Can you work these out from the drawing? Everything is in mm from the part's minimum corner. A direction names the side the tool comes from. Round coordinates to 2 decimals unless told otherwise and drop trailing zeros. Loops run counter-clockwise (first coordinate to the right, second up) from the corner with the lowest first, then second, coordinate; pieces in that order, holes last. Notation, with made-up numbers: M -22.75,75.25 L -3.75,75.25 A32 cw -3.75,103.25 Z; hole C -4.75,11 d1. An arc over 180 degrees is marked long. Use a Markdown table: item, result.
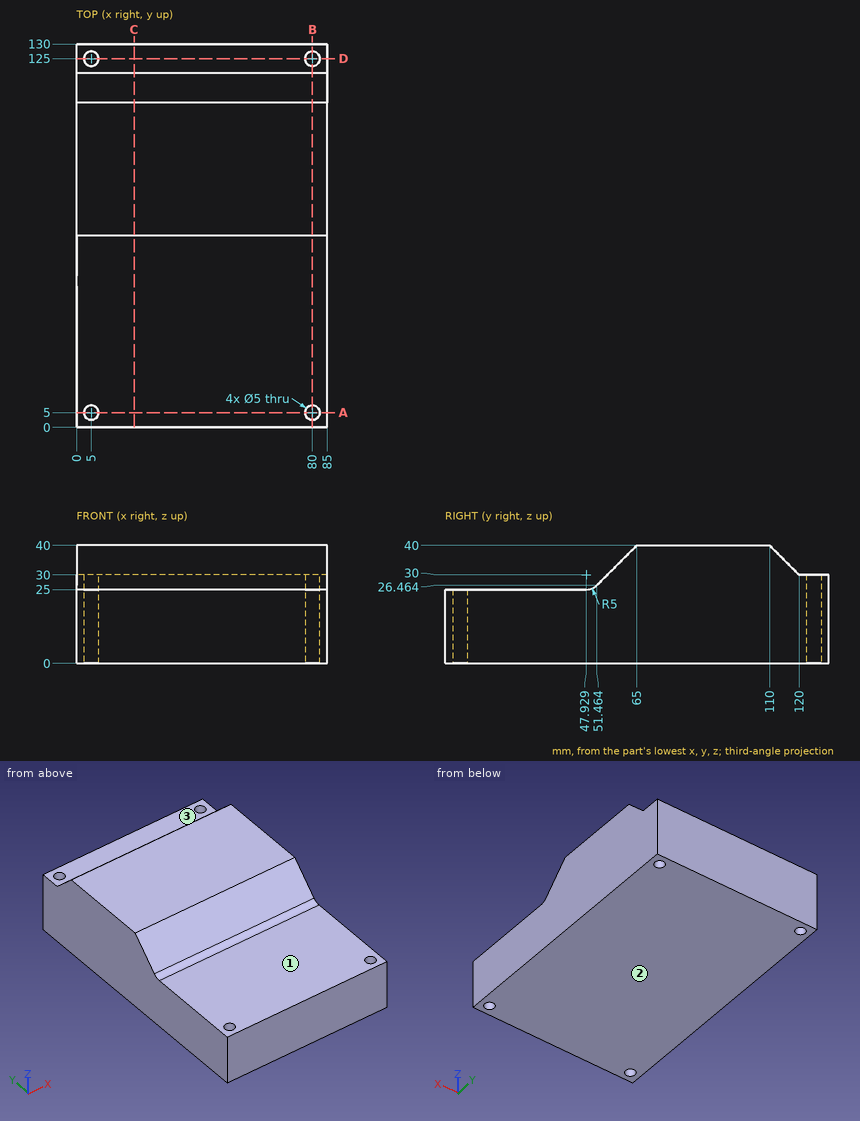
Q1. I need wall thicknesses on line 1 (Y direction, x = 80, z = 21); line 2 (X direction, y = 125, z = 16.5); line 3 (Y direction, x = 78.5, z = 19.5). Which ranges of each line are inside material? Lowest first, please. Write a range as from..to.
Return value:
| item | result |
|---|---|
| line 1 | y = 0..2.5, 7.5..122.5, 127.5..130 |
| line 2 | x = 0..2.5, 7.5..77.5, 82.5..85 |
| line 3 | y = 0..3, 7..123, 127..130 |
Q2. Imagine slicing it at C-C, the plane x = 19.5. Please give me the cut outline in (y, z) (1 decimal).
Return value:
| item | result |
|---|---|
| outline | M 0,0 L 130,0 L 130,30 L 120,30 L 110,40 L 65,40 L 51.5,26.5 A5 cw 47.9,25 L 0,25 Z |
Q3. For the marked faces 1, 2 and 3, which set-ups out of +Z, -Z, +X, -X, +Y, -Y let a thin tool reach every point of the face, with its end or its side?
Return value:
| item | result |
|---|---|
| face 1 | +Z, +X, -X, -Y |
| face 2 | -Z, +X, -X, +Y, -Y |
| face 3 | +Z, +X, -X, +Y |
Q4. Imagine slicing it at D-D, the plane y = 125. Please give me the cut outline in (x, z).
Return value:
| item | result |
|---|---|
| outline | M 0,0 L 2.5,0 L 2.5,30 L 0,30 Z; M 7.5,0 L 77.5,0 L 77.5,30 L 7.5,30 Z; M 82.5,0 L 85,0 L 85,30 L 82.5,30 Z |
Q5. Imagine slicing it at B-B, the plane x = 80. Please give me the cut outline in (y, z) (1 decimal).
Return value:
| item | result |
|---|---|
| outline | M 0,0 L 2.5,0 L 2.5,25 L 0,25 Z; M 7.5,0 L 122.5,0 L 122.5,30 L 120,30 L 110,40 L 65,40 L 51.5,26.5 A5 cw 47.9,25 L 7.5,25 Z; M 127.5,0 L 130,0 L 130,30 L 127.5,30 Z |
Q6. Imagine slicing it at A-A, the plane y = 5. Please give me the cut outline in (x, z), then the cut area to 4 significant figures.
Return value:
| item | result |
|---|---|
| outline | M 0,0 L 2.5,0 L 2.5,25 L 0,25 Z; M 7.5,0 L 77.5,0 L 77.5,25 L 7.5,25 Z; M 82.5,0 L 85,0 L 85,25 L 82.5,25 Z |
| area | 1,875 mm^2 |
Q7. Will these pins go through, and if not, where does the flat tip stop? P1, Ø4, axis at x = 80, y = 125, coming from the +Z side; P2, Ø11, axis at x = 34, y = 124, coming from the +Z side; P3, Ø6.5, axis at x = 80, y = 5, coming from the +Z side; P4, Ø8, axis at x = 5, y = 125, coming from the +Z side.
Return value:
| item | result |
|---|---|
| P1 | passes through |
| P2 | stops at z = 31.5 |
| P3 | stops at z = 25 |
| P4 | stops at z = 30 |
